from build123d import *

# Parameters (mm, degrees)
BOSS_EXTRUDE1_DEPTH     = 6
CUT_EXTRUDE1_DEPTH      = 43.812285079
CUT_EXTRUDE2_DEPTH      = 43.812285079
F_1_4_28_TAPPED_HOLE1_D = 5.4102


with BuildPart() as part:
    # Sketch1 → Boss-Extrude1 (new body)
    with BuildSketch(Plane(origin=(0, 0, 0), x_dir=(1, 0, 0), z_dir=(0, 1, 0))):
        with BuildLine():
            ThreePointArc((-43.5, 11.4), (-45.403805922, 15.996194078), (-50, 17.9))
            Line((-50, 17.9), (-50, 70))
            ThreePointArc((-50, 70), (-41.213203436, 91.213203436), (-20, 100))
            Line((-20, 100), (-15.5, 100))
            ThreePointArc((-15.5, 100), (-13.378679656, 100.878679656), (-12.5, 103))
            Line((-12.5, 103), (-12.5, 109.304760106))
            ThreePointArc((-12.5, 109.304760106), (0, 117), (12.5, 109.304760106))
            Line((12.5, 109.304760106), (12.5, 103))
            ThreePointArc((12.5, 103), (13.378679656, 100.878679656), (15.5, 100))
            Line((15.5, 100), (20, 100))
            ThreePointArc((20, 100), (41.213203436, 91.213203436), (50, 70))
            Line((50, 70), (50, 17.9))
            ThreePointArc((50, 17.9), (45.403805922, 15.996194078), (43.5, 11.4))
            Line((43.5, 11.4), (43.5, 5.221716559))
            Line((43.5, 5.221716559), (0, 0))
            Line((0, 0), (-43.5, 5.221716559))
            Line((-43.5, 5.221716559), (-43.5, 11.4))
        make_face()
        with BuildLine():
            ThreePointArc((2.1, 111), (0, 113.1), (-2.1, 111))
            Line((-2.1, 111), (-2.1, 108))
            ThreePointArc((-2.1, 108), (0, 105.9), (2.1, 108))
            Line((2.1, 108), (2.1, 111))
        make_face(mode=Mode.SUBTRACT)
    extrude(amount=BOSS_EXTRUDE1_DEPTH)

    # Sketch2 → Cut-Extrude1 (cut, along a direction that is not the sketch's normal)
    with BuildSketch(Plane(origin=(0, 0, 0), x_dir=(0, 0, -1), z_dir=(1, 0, 0))):
        Polygon((5.640200242, 6), (0, 0.400000131), (0, 6), align=None)
    extrude(amount=CUT_EXTRUDE1_DEPTH, dir=(0.9928722028940861, 0, -0.11918384420820177), mode=Mode.SUBTRACT)

    # Sketch2<2> → Cut-Extrude2 (cut, along a direction that is not the sketch's normal)
    with BuildSketch(Plane(origin=(0, 0, 0), x_dir=(0, 0, -1), z_dir=(1, 0, 0))):
        Polygon((5.640200242, 6), (0, 0.400000131), (0, 6), align=None)
    extrude(amount=-CUT_EXTRUDE2_DEPTH, dir=(0.9928722028940861, 0, 0.11918384420820147), mode=Mode.SUBTRACT)

    # 1/4-28 Tapped Hole1 (through all)
    with Locations(Plane(origin=(0, 6, 0), x_dir=(1, 0, 0), z_dir=(0, 1, 0))):
        with Locations((-25.4, 75.8), (25.4, 75.8), (25.4, 25), (-25.4, 25)):
            Hole(F_1_4_28_TAPPED_HOLE1_D / 2)


solid = part.part
Geometry: final body of the model. Coordinates: model frame, mm. A direction names the side the tool comes from. Round coordinates to 2 decimals unless told otherwise and drop trailing zeros. Loops run counter-clockwise (first coordinate to the right, second up) from the corner with the lowest first, then second, coordinate; pieces in that order, holes last.
Q1. Pull-direction query (X, two-part tool) for faces 1 (the cylindrical face through (0, 3, -113.1)), 2 (the cylindrical face through (-22.698, 2.958, -25.119)), 3 (the flat face through (-21.446, 3.276, -5.471)), 4 (the cylindrical face through (0, 3, -117)); classes: released by +X, released by -X, zero draft, split by the parting line, or undercut.
Q2. Access query for faces 5 (the flat face through (-18, 3, -100)), 6 (the flat face through (18, 3, -100)), 7 (the flat face through (-43.5, 2, -9)). Directions: +Z, -Z, +X, -X, +Y, -Y. A direction counts if a zero-diameter tool reaches every point of the face in a straight line with its end or side. Return the directions, or none.
Q3. Section B-B on y = 4.2. Return loops of the section in (x, z), plus the area to 3 significant figures.
Q4. Material intervals for L1, parallel to X at y = 2.6, z = -75.8; L2, parallel to X at y = 3.6, z = -25; L3, parallel to Z at x = 25.4, y = 3.3, sorted ascending.
Q5. Section C-C on x = -25.4. Return loops of the section in (y, z), plus the area to 3 significant figures.
Q6. Section A-A on z = -75.8. Return loops of the section in (x, y).
Q7. Pin query (flat end, axial travel): P1, Ø3.5, axis at x = -18, y = 3.5, coming from the -Z side; P2, Ø3, axis at y = 1.5, z = -106.5, coming from the +X side; P3, Ø1.5, axis at y = 4, z = -85.5, coming from the -X side; P4, Ø7, axis at x = 25.4, z = -25, coming from the -Y side. Return the tip coordinate at first contact, or that it passes through.
Q8. Section D-D on x = -9. Return loops of the section in (y, z), plus the area to 3 significant figures.
Evaluation:
1. face 1: undercut
1. face 2: undercut
1. face 3: released by -X
1. face 4: split by the parting line
2. face 5: -Z, -X, +Y, -Y
2. face 6: -Z, +X, +Y, -Y
2. face 7: +Z, -X, +Y, -Y
3. outline: (-50, -70) arc R30 ccw to (-20, -100) - (-15.5, -100) arc R3 cw to (-12.5, -103) - (-12.5, -109.3) arc R14 ccw to (12.5, -109.3) - (12.5, -103) arc R3 cw to (15.5, -100) - (20, -100) arc R30 ccw to (50, -70) - (50, -17.9) arc R6.5 cw to (43.5, -11.4) - (43.5, -9.05) - (0, -3.83) - (-43.5, -9.05) - (-43.5, -11.4) arc R6.5 cw to (-50, -17.9) - close; hole circle Ø5.41 at (-25.4, -75.8); hole circle Ø5.41 at (-25.4, -25); hole (-2.1, -111) arc R2.1 ccw to (2.1, -111) - (2.1, -108) arc R2.1 ccw to (-2.1, -108) - close; hole circle Ø5.41 at (25.4, -75.8); hole circle Ø5.41 at (25.4, -25)
3. area: 9,090 mm2
4. L1: x = -49.43 to -28.11, -22.69 to 22.69, 28.11 to 49.43
4. L2: x = -50 to -28.11, -22.69 to 22.69, 28.11 to 50
4. L3: z = -99.51 to -78.51, -73.09 to -27.71, -22.29 to -5.97
5. outline: (0, -99.51) - (6, -99.51) - (6, -78.51) - (0, -78.51) - close; (0, -73.09) - (6, -73.09) - (6, -27.71) - (0, -27.71) - close; (0, -22.29) - (6, -22.29) - (6, -8.69) - (0.4, -3.05) - (0, -3.05) - close
5. area: 498 mm2
6. outline: (-49.43, 0) - (-28.11, 0) - (-28.11, 6) - (-49.43, 6) - close; (-22.69, 0) - (22.69, 0) - (22.69, 6) - (-22.69, 6) - close; (28.11, 0) - (49.43, 0) - (49.43, 6) - (28.11, 6) - close
7. P1: stops at z = -100
7. P2: stops at x = 12.5
7. P3: stops at x = -46.12
7. P4: stops at y = 0
8. outline: (0, -113.72) - (6, -113.72) - (6, -6.72) - (0.4, -1.08) - (0, -1.08) - close
8. area: 660 mm2
